Can you work these out from the model? Positions are in its coordinate system, mm. Face numbers are marked on the shaded views. A direction names the side the tool comes from. Coordinates: 2 decimals unless noted, no trailing zeros. Order: outer loops, then holes, each group sorted by start corner. A loop starts at its lowest first (then second) coordinate and runs counter-clockwise, first axis right, second up. Notation, with made-up numbers: (38, 58) -> (56, 58) arc R22 ccw to (56, 64) -> close; hole circle Ø2 at (67.5, 47). An arc over 180 degrees is marked (long way). Answer in a Markdown table with one row per item. Add a question column.
1. On a 3-axis mill with a long thin cutter (end or side, diameter ignored), from which of +Z, -Z, +X, -X, +Y, -Y can I reach the whole of each face in a straight line? I mean the marked faces 1, 2 and 3. Say none if no direction works.
2. Imagine slicing it at D-D on x = -535.7. Write out the boundary of the cut face in (y, z).
3. Imagine slicing it at A-A on y = 224.6. Write out the boundary of the cut face in (x, z).
4. Imagine slicing it at B-B on x = -536.65. Write out the boundary of the cut face in (y, z), plus the area to 3 significant figures.
5. Will these pins go through, and if not, where does the flat tip stop? pin 1 (1 mm diameter, centred on y = 224, z = 4.5, fed in from -X); pin 2 (1.5 mm diameter, centred on y = 224, z = 4, fed in from -X); pin 3 (3 mm diameter, centred on x = -538.5, y = 223.5, fed in from -Z); pin 4 (1 mm diameter, centred on x = -538.5, z = 4.5, fed in from +Y).
6. If I drill on line 1 along Z through (x, y) = (-536.05, 224.7); line 2 along X through (y, z) = (226.7, 3.5); line 3 along Y through (x, z) = (-538.45, 4.75), over which ranges is the centre line in solid material (lowest first)? Write a range as [from, to].
7. Imagine slicing it at C-C on z = 2.5. Write out the boundary of the cut face in (x, y).
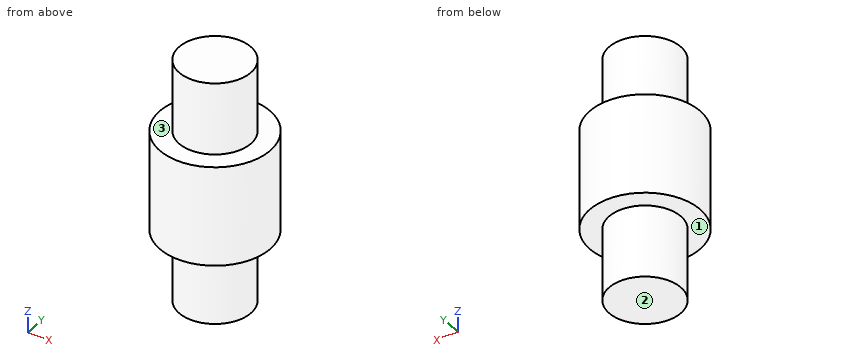
Autodesk Inventor part; units mm, degrees
ref_plane "YZ Plane" through (0, 0, 0) normal (1, 0, 0) x (0, 1, 0)
ref_plane "XZ Plane" through (0, 0, 0) normal (0, 1, 0) x (-1, 0, 0)
ref_plane "XY Plane" through (0, 0, 0) normal (0, 0, 1) x (1, 0, 0)
sketch "Sketch1" plane through (0, 0, 0) normal (0, 0, 1) x (1, 0, 0)
  circle A0 centre (-537.6416, 225.4624) radius 2.54
  point P0 (0, 0)
  dimension "d0" = 5.08
extrude "Extrusion1" add sketch "Sketch1" along normal blind 4.572
sketch "Sketch2" plane through (-537.6416, 225.4624, 4.572) normal (0, 0, 1) x (1, 0, 0)
  circle A0 centre (0, 0) radius 2.54
  circle A1 centre (0, 0) radius 1.651
  point P0 (537.6416, -225.4624)
  dimension "d3" = 3.302
extrude "Extrusion2" add sketch "Sketch2" along normal blind 3.302 contours A1
sketch "Sketch3" plane through (-537.6416, 225.4624, 0) normal (0, 0, -1) x (-1, 0, 0)
  circle A0 centre (0, 0) radius 2.54
  circle A1 centre (0, 0) radius 1.651
  point P0 (-537.6416, -225.4624)
  dimension "d6" = 3.302
extrude "Extrusion3" add sketch "Sketch3" along normal blind 3.302 contours A1
properties part number "chain_axel"
Answers follow:
| question | item | result |
|---|---|---|
| 1 | face 1 | -Z |
| 1 | face 2 | -Z, +X, -X, +Y, -Y |
| 1 | face 3 | +Z |
| 2 | outline | (223.82, 0) -> (227.1, 0) -> (227.1, 4.57) -> (223.82, 4.57) -> close |
| 3 | outline | (-540.03, 0) -> (-539.05, 0) -> (-539.05, -3.3) -> (-536.23, -3.3) -> (-536.23, 0) -> (-535.25, 0) -> (-535.25, 4.57) -> (-536.23, 4.57) -> (-536.23, 7.87) -> (-539.05, 7.87) -> (-539.05, 4.57) -> (-540.03, 4.57) -> close |
| 4 | outline | (223.12, 0) -> (224.14, 0) -> (224.14, -3.3) -> (226.78, -3.3) -> (226.78, 0) -> (227.8, 0) -> (227.8, 4.57) -> (226.78, 4.57) -> (226.78, 7.87) -> (224.14, 7.87) -> (224.14, 4.57) -> (223.12, 4.57) -> close |
| 4 | area | 38.8 mm² |
| 5 | pin 1 | stops at x = -539.99 |
| 5 | pin 2 | stops at x = -540.08 |
| 5 | pin 3 | stops at z = -3.3 |
| 5 | pin 4 | stops at y = 227.98 |
| 6 | line 1 | z = [0, 4.57] |
| 6 | line 2 | x = [-539.86, -535.42] |
| 6 | line 3 | y = [224.02, 226.9] |
| 7 | outline | circle Ø5.08 at (-537.64, 225.46) |
